from build123d import *

# Parameters (mm, degrees)
ESQUISSE1_W             = 14
ESQUISSE1_H             = 7.9
ESQUISSE1_W_2           = 8
BOSS_EXTRU_1_DEPTH      = 5.3
ESQUISSE1_4_W           = 8
ESQUISSE1_4_H           = 7.9
BOSS_EXTRU_2_DEPTH      = 7.3
ESQUISSE2_OUTSIDE_W     = 28.898
ESQUISSE2_OUTSIDE_H     = 14.798
ENL_V_MAT_EXTRU_2_DEPTH = 2
D_GAGEMENT_M31_D        = 3.2
CONG_1_R                = 1
ESQUISSE5_W             = 6
ESQUISSE5_H             = 4.8
BOSS_EXTRU_3_DEPTH      = 1.2
ESQUISSE6_R             = 1.5
BOSS_EXTRU_4_DEPTH      = 15


with BuildPart() as part:
    # Esquisse1 → Boss.-Extru.1 (new body)
    with BuildSketch(Plane(origin=(0, 0, 0), x_dir=(1, 0, 0), z_dir=(0, 1, 0))):
        with Locations((11, 0)):
            Rectangle(ESQUISSE1_W, ESQUISSE1_H)
        Rectangle(ESQUISSE1_W_2, ESQUISSE1_H)
    extrude(amount=BOSS_EXTRU_1_DEPTH)

    # Esquisse1<4> → Boss.-Extru.2 (add)
    with BuildSketch(Plane(origin=(0, 0, 0), x_dir=(1, 0, 0), z_dir=(0, 1, 0))):
        Rectangle(ESQUISSE1_4_W, ESQUISSE1_4_H)
    extrude(amount=BOSS_EXTRU_2_DEPTH)

    # Esquisse2 outside → Enlèv. mat.-Extru.2 (cut)
    with BuildSketch(Plane(origin=(0, 7.3, 0), x_dir=(1, 0, 0), z_dir=(0, 1, 0))):
        with Locations((7, 0)):
            Rectangle(ESQUISSE2_OUTSIDE_W, ESQUISSE2_OUTSIDE_H)
        with BuildLine():
            Line((4, -0.95), (4, 0.95))
            ThreePointArc((4, 0.95), (3.121320344, 3.071320344), (1, 3.95))
            Line((1, 3.95), (-1, 3.95))
            ThreePointArc((-1, 3.95), (-3.121320344, 3.071320344), (-4, 0.95))
            Line((-4, 0.95), (-4, -0.95))
            ThreePointArc((-4, -0.95), (-3.121320344, -3.071320344), (-1, -3.95))
            Line((-1, -3.95), (1, -3.95))
            ThreePointArc((1, -3.95), (3.121320344, -3.071320344), (4, -0.95))
        make_face(mode=Mode.SUBTRACT)
    extrude(amount=-ENL_V_MAT_EXTRU_2_DEPTH, mode=Mode.SUBTRACT)

    # Dégagement M31 (through all)
    with Locations(Plane(origin=(0, 5.3, 0), x_dir=(1, 0, 0), z_dir=(0, 1, 0))):
        with Locations((11.7, 0)):
            Hole(D_GAGEMENT_M31_D / 2)

    # Congé1
    cong_1_edges = [part.edges().sort_by_distance(p)[0] for p in [
        (-4, 2.65, 3.95),
        (-4, 2.65, -3.95),
    ]]
    fillet(cong_1_edges, radius=CONG_1_R)

    # Esquisse5 → Boss.-Extru.3 (add)
    with BuildSketch(Plane(origin=(18, 0, 0), x_dir=(0, 0, -1), z_dir=(1, 0, 0))):
        with Locations((0, 2.4)):
            Rectangle(ESQUISSE5_W, ESQUISSE5_H)
    extrude(amount=BOSS_EXTRU_3_DEPTH)

    # Esquisse6 → Boss.-Extru.4 (add)
    with BuildSketch(Plane(origin=(19.2, 0, 0), x_dir=(0, 0, -1), z_dir=(1, 0, 0))):
        with Locations((0, 2.7)):
            Circle(ESQUISSE6_R)
    extrude(amount=BOSS_EXTRU_4_DEPTH)


solid = part.part
Read the model definition and answer for the solid it produces. Units are mm, in the model's axes. A direction names the side the tool comes from. Coordinates: 2 decimals unless noted, no trailing zeros. Loops run counter-clockwise (first coordinate to the right, second up) from the corner with the lowest first, then second, coordinate; pieces in that order, holes last. Notation, with made-up numbers: (76, 44.5) - (97, 44.5) arc R10 ccw to (97, 53.5) - close; hole circle Ø3 at (-35.75, 23.25). An arc over 180 degrees is marked (long way). Answer in a Markdown table with one row per item.
Q1. Find section D-D on y = 5.75. Write down the section's boundary in (x, z), plus the area to 3 significant figures.
Here are the results:
| item | result |
|---|---|
| outline | (-4, -0.95) arc R3 ccw to (-1, -3.95) - (1, -3.95) arc R3 ccw to (4, -0.95) - (4, 0.95) arc R3 ccw to (1, 3.95) - (-1, 3.95) arc R3 ccw to (-4, 0.95) - close |
| area | 55.5 mm^2 |
Q2. Find section C-C on z = 0. Write down the section's boundary in (x, y), plus the area to 3 significant figures.
Here are the results:
| item | result |
|---|---|
| outline | (-4, 0) - (10.1, 0) - (10.1, 5.3) - (4, 5.3) - (4, 7.3) - (-4, 7.3) - close; (13.3, 0) - (19.2, 0) - (19.2, 1.2) - (34.2, 1.2) - (34.2, 4.2) - (19.2, 4.2) - (19.2, 4.8) - (18, 4.8) - (18, 5.3) - (13.3, 5.3) - close |
| area | 166 mm^2 |
Q3. The mould has two halves that part along X. Classify faces 5 (the cylindrical face through (-3.14, 6.31, 3.05)), 6 (the cylindrical face through (10.174, 2.613, -0.481)), 7 (the flat face through (9, 5.3, 0)): pulls with the +X half, pulls with the -X half, needs draft (parallel to the pull), parting line crosses it, or undercut.
Here are the results:
| item | result |
|---|---|
| face 5 | pulls with the -X half |
| face 6 | undercut |
| face 7 | needs draft |
Q4. Given P1, Ø2, axis at x = 29, y = 5.5, coming from the +Z side; P2, Ø1.5, axis at x = 6.5, z = 2.5, coming from the +Y side; P3, Ø1.5, axis at x = 19.5, y = 3, coming from the -Z side; P4, Ø1.5, axis at x = 28.5, y = 1, coming from the -Z side, each flat-ended and moving along its own axis, determine where each tip first touches the part or whether it passes through.
Here are the results:
| item | result |
|---|---|
| P1 | passes through |
| P2 | stops at y = 5.3 |
| P3 | stops at z = -3 |
| P4 | stops at z = -1.16 |
Q5. For faces 1 (the flat face through (-3.285, 5.3, -3.124)), 2 (the cylindrical face through (26.595, 4.187, 0.195)), 3 (the flat face through (4, 6, 0)), 4 (the flat face through (19, 2, -3)), determine the directions among +Z, -Z, +X, -X, +Y, -Y from which every point of the face is accessible in a straight line to the end or side of a thin tool.
Here are the results:
| item | result |
|---|---|
| face 1 | -Z, -X, +Y |
| face 2 | +X |
| face 3 | +Z, -Z, +X, +Y |
| face 4 | -Z, +X, +Y, -Y |
Q6. Find section B-B on y = 0.5. Write down the section's boundary in (x, z).
Here are the results:
| item | result |
|---|---|
| outline | (-4, -2.95) arc R1 ccw to (-3, -3.95) - (18, -3.95) - (18, -3) - (19.2, -3) - (19.2, 3) - (18, 3) - (18, 3.95) - (-3, 3.95) arc R1 ccw to (-4, 2.95) - close; hole circle Ø3.2 at (11.7, 0) |
Q7. Find section A-A on x = 11.7. Write down the section's boundary in (y, z), plus the area to 3 significant figures.
Here are the results:
| item | result |
|---|---|
| outline | (0, -3.95) - (5.3, -3.95) - (5.3, -1.6) - (0, -1.6) - close; (0, 1.6) - (5.3, 1.6) - (5.3, 3.95) - (0, 3.95) - close |
| area | 24.9 mm^2 |
Q8. Straight lines are drawn through the part: line 1 along Z through (x, y) = (11.7, 4); line 2 along Y through (x, z) = (7.5, 0.75); line 3 along X through (y, z) = (6.25, -0.75). For each, find the intervals that lie inside material, in ascending order. Write a range as [from, to].
Here are the results:
| item | result |
|---|---|
| line 1 | z = [-3.95, -1.6], [1.6, 3.95] |
| line 2 | y = [0, 5.3] |
| line 3 | x = [-4, 4] |
